Check sheet for the modelled part. Datum: model origin and axes. Units: mm. A direction names the side the tool comes from. Round coordinates to 2 decimals unless told otherwise and drop trailing zeros. Write each loop counter-clockwise with the first axis right and the second up, starting at its lowest first coordinate (ties: lowest second). Pieces come first, ordered by that corner, then holes. Notation, with made-up numbers: (30.5, 34.5) -> (88.5, 34.5) arc R6 cw to (88.5, 39.5) -> close; hole circle Ø3 at (38, 74). An arc over 180 degrees is marked (long way). Write item = value, one per line.
Autodesk Inventor part; units mm, degrees
ref_plane "YZ Plane" through (0, 0, 0) normal (1, 0, 0) x (0, 1, 0)
ref_plane "XZ Plane" through (0, 0, 0) normal (0, 1, 0) x (-1, 0, 0)
ref_plane "XY Plane" through (0, 0, 0) normal (0, 0, 1) x (1, 0, 0)
sketch "スケッチ1" plane through (0, 0, 0) normal (0, 0, 1) x (1, 0, 0)
  circle A0 centre (0, 0) radius 9
  circle A1 centre (0, 0) radius 1
  dimension "d0" = 18
  dimension "d3" = 2
extrude "押し出し1" add sketch "スケッチ1" along normal mid plane 20
sketch "スケッチ2" plane through (0, 0, -10) normal (0, 0, -1) x (-1, 0, 0)
  line L0 (-1, 10.2383) -> (1, 10.2383)
  line L1 (1, 10.2383) -> (1, -10.4548)
  line L2 (1, -10.4548) -> (-1, -10.4548)
  line L3 (-1, -10.4548) -> (-1, 10.2383)
  point P0 (0, 0)
  point P1 (0, -10.4548)
  dimension "d4" = 2
extrude "押し出し2" cut sketch "スケッチ2" against normal blind 3
thread "ねじ1"
sketch "スケッチ3" plane through (0, 0, 10) normal (0, 0, 1) x (1, 0, 0)
  point P0 (0, 0)
sketch "スケッチ4" plane through (0, 0, 10) normal (0, 0, 1) x (1, 0, 0)
  circle A0 centre (0, 0) radius 6.5
  dimension "d9" = 13
extrude "押し出し3" cut sketch "スケッチ4" against normal blind 12
properties part number "rod330_end_screw" material "ステンレス鋼"
(1) Sectioned sample at C-C on y = 6. Enter the section's corners in (x, z).
Worked answers:
outline = (-6.71, -10) -> (-1, -10) -> (-1, -7) -> (1, -7) -> (1, -10) -> (6.71, -10) -> (6.71, 10) -> (2.5, 10) -> (2.5, -2) -> (-2.5, -2) -> (-2.5, 10) -> (-6.71, 10) -> close
(2) Sectioned sample at B-B on z = -5.5. Enter the section's corners in (x, y), then the cut area to 3 significant figures.
Worked answers:
outline = circle Ø18 at (0, 0); hole circle Ø2 at (0, 0)
area = 251 mm²
(3) Access from +Z, -Z, +X, -X, +Y, -Y to the whole of each face (thin tool, end or side, straight path). Record for faces 1 (the cylindrical face through (-5.158, -3.955, 4.084)), 2 (the flat face through (0, -4, -7)), 3 (the flat face through (4, 0, -10)).
Worked answers:
face_1 = +Z
face_2 = -Z, +Y, -Y
face_3 = -Z, +X, -X, +Y, -Y
(4) Sectioned sample at A-A on x = 0. Enter the section's corners in (y, z).
Worked answers:
outline = (-9, -7) -> (-1, -7) -> (-1, -2) -> (-6.5, -2) -> (-6.5, 10) -> (-9, 10) -> close; (1, -7) -> (9, -7) -> (9, 10) -> (6.5, 10) -> (6.5, -2) -> (1, -2) -> close
(5) Release check for a two-part mould opening along Y. For faces 4 (the cylindrical face through (-1.172, -8.923, -0.14)), 5 (the cylindrical face through (0, -1, -4)), 6 (the flat face through (0, 5, -7)) record: pulls with the +Y half, pulls with the -Y half, needs draft (parallel to the pull), parting line crosses it, or undercut.
Worked answers:
face_4 = parting line crosses it
face_5 = undercut
face_6 = needs draft
(6) Material ranges on L1, parallel to Y at x = 0, z = 1; L2, parallel to X at y = 0, z = -5.2, recorded low to high. Write a range as [from, to].
Worked answers:
L1 = [-9, -6.5], [6.5, 9]
L2 = [-9, -1], [1, 9]
(7) Go/stop test with flat-tipped pins: P1, Ø4, axis at x = -1.5, y = -0.5, coming from the +Z side; P2, Ø6, axis at y = -5, z = 7.5, coming from the -X side; P3, Ø6, axis at x = -2.5, y = -3.5, coming from the +Z side; P4, Ø1.5, axis at x = 5, z = 6, coming from the -Y side. Record where each tip stops, or that it passes through.
Worked answers:
P1 = -2
P2 = -8.77
P3 = 10
P4 = -7.93
(8) Sectioned sample at D-D on x = 5.75. Enter the section's corners in (y, z).
Worked answers:
outline = (-6.92, -10) -> (6.92, -10) -> (6.92, 10) -> (3.03, 10) -> (3.03, -2) -> (-3.03, -2) -> (-3.03, 10) -> (-6.92, 10) -> close
